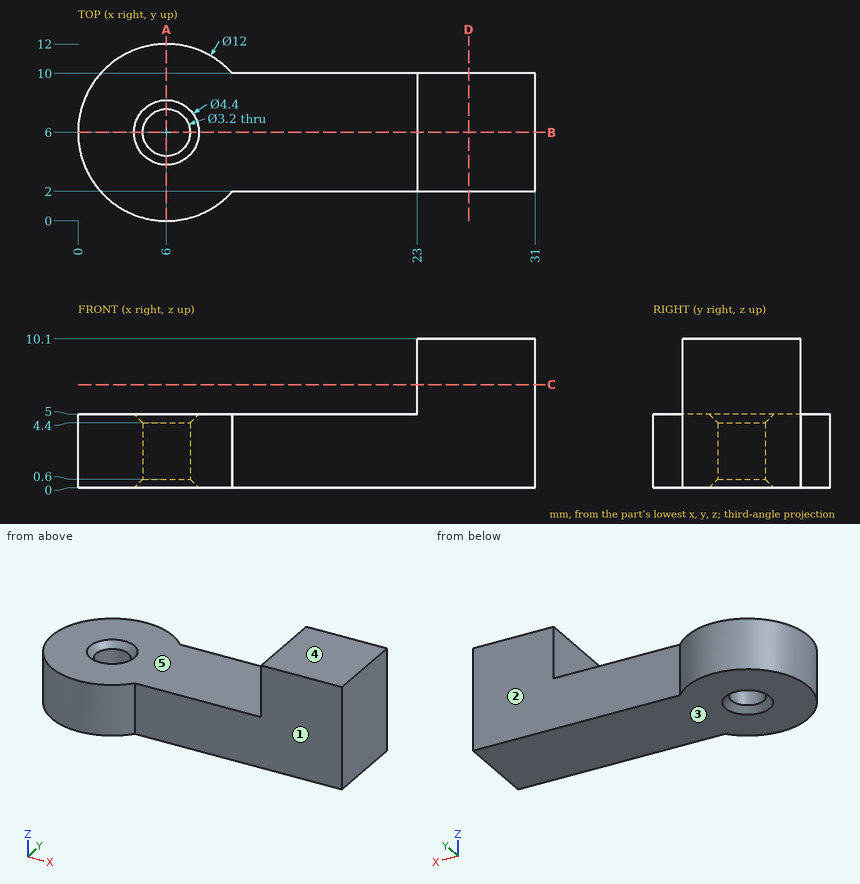
Check sheet for the drawn part. Datum: minimum x, y, z corner. Units: mm. A direction names the side the tool comes from. Give positions to 0.01 mm unless a question says otherwise; leave off trailing zeros. Order: outer loops, then holes, each group sorted by start corner. A loop starts at its lowest first (then second) coordinate and runs counter-clockwise, first axis right, second up. Notation, with made-up numbers: (-27.75, 33.25) -> (16.25, 33.25) arc R27 cw to (16.25, 53.25) -> close; hole circle Ø11 at (48.5, 21.25). An arc over 180 degrees is marked (long way). One line per item, written item: value.
(1) Scan lines: line 1 along Y through (x, z) = (6, 3.05); line 2 along X through (y, z) = (6, 1.75); line 3 along Z through (x, y) = (17.5, 3.5). Record each from-to range of solid material in increasing order. Write a range as [from, to].
Final values:
line 1: [0, 4.4], [7.6, 12]
line 2: [0, 4.4], [7.6, 31]
line 3: [0, 5]
(2) Sectioned sample at D-D on x = 26.5. Record the cut outline in (y, z), then the cut area to 3 significant figures.
Final values:
outline: (2, 0) -> (10, 0) -> (10, 10.1) -> (2, 10.1) -> close
area: 80.8 mm^2
(3) Sectioned sample at C-C on z = 7. Record the cut outline in (x, y).
Final values:
outline: (23, 2) -> (31, 2) -> (31, 10) -> (23, 10) -> close
(4) Tool access check on the marked faces 1, 2, 3, 4 and 5. Record the directions out of +Z, -Z, +X, -X, +Y, -Y that give a thin tool (end or side, any length) a straight path to the whole face; none if there is none.
Final values:
face 1: +Z, -Z, +X, -Y
face 2: +Z, -Z, +X, +Y
face 3: -Z, +X, -X, +Y, -Y
face 4: +Z, +X, -X, +Y, -Y
face 5: +Z, -X, +Y, -Y
(5) Sectioned sample at A-A on x = 6. Record the cut outline in (y, z), then the cut area to 3 significant figures.
Final values:
outline: (0, 0) -> (3.8, 0) -> (4.4, 0.6) -> (4.4, 4.4) -> (3.8, 5) -> (0, 5) -> close; (7.6, 0.6) -> (8.2, 0) -> (12, 0) -> (12, 5) -> (8.2, 5) -> (7.6, 4.4) -> close
area: 43.3 mm^2
(6) Sectioned sample at B-B on y = 6. Record the cut outline in (x, z), then the cut area to 3 significant figures.
Final values:
outline: (0, 0) -> (3.8, 0) -> (4.4, 0.6) -> (4.4, 4.4) -> (3.8, 5) -> (0, 5) -> close; (7.6, 0.6) -> (8.2, 0) -> (31, 0) -> (31, 10.1) -> (23, 10.1) -> (23, 5) -> (8.2, 5) -> (7.6, 4.4) -> close
area: 179 mm^2
(7) Gauge pin test, flat ends, axial feed: pin 1 (5 mm diameter, centred on x = 12, z = 5, fed in from -Y); pin 2 (5 mm diameter, centred on x = 23.5, z = 3.5, fed in from -Y); pin 3 (5 mm diameter, centred on x = 25.5, z = 4.5, fed in from +Y); pin 4 (2.5 mm diameter, centred on x = 6, y = 6, fed in from -Z). Record the tip position at first contact, or that the pin passes through.
Final values:
pin 1: y = 1.13
pin 2: y = 2
pin 3: y = 10
pin 4: through
